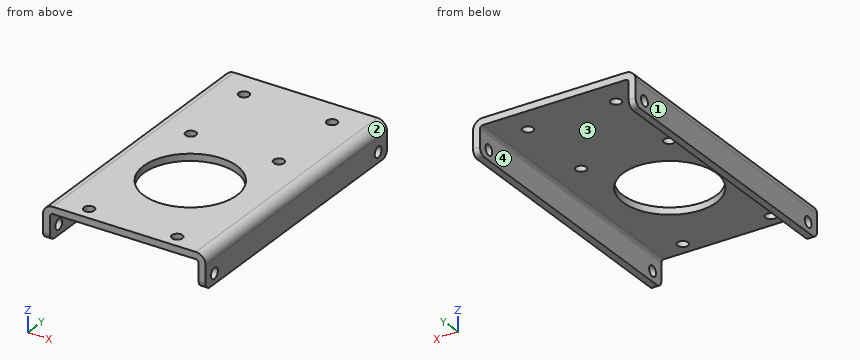
from build123d import *

# Parameters (mm, degrees)
SKETCH1_W                      = 76.2
SKETCH1_H                      = 130.175
BASE_FLANGE1_DEPTH             = 3.2639
EDGE_FLANGE1_STRIP_W           = 15.5956
EDGE_FLANGE1_STRIP_H           = 3.2639
EDGE_FLANGE1_STRIP_CUT_DEPTH   = 130.175
EDGE_FLANGE1_STRIP_2_W         = 15.5956
EDGE_FLANGE1_STRIP_2_H         = 3.2639
EDGE_FLANGE1_STRIP_CUT_2_DEPTH = 130.175
EDGE_FLANGE1_DEPTH             = 130.175
EDGE_FLANGE1_BEND_DEPTH        = 130.175
F_10_0_1935_DIAMETER_HOLE1_D   = 4.9149
SKETCH32_R                     = 21.87575
CUT_EXTRUDE1_DEPTH             = 93.055303045
F_10_0_1935_DIAMETER_HOLE2_D   = 4.9149
FILLET1_R                      = 3.175
F_10_0_1935_DIAMETER_HOLE3_D   = 4.9149


# Sheet-metal steps are written as plain solids
with BuildPart() as part:
    # Sketch1 → Base-Flange1 (new body)
    with BuildSketch(Plane.XY):
        with Locations((0, 17.758918)):
            Rectangle(SKETCH1_W, SKETCH1_H)
    extrude(amount=-BASE_FLANGE1_DEPTH)

    # Edge-Flange1 strip (across the edge) → Edge-Flange1 strip cut (cut)
    with BuildSketch(Plane(origin=(38.1, 82.846418, -3.2639), x_dir=(-1, 0, 0), z_dir=(0, -1, 0))):
        with Locations((-3.2639, -1.63195)):
            Rectangle(EDGE_FLANGE1_STRIP_W, EDGE_FLANGE1_STRIP_H)
    extrude(amount=EDGE_FLANGE1_STRIP_CUT_DEPTH, mode=Mode.SUBTRACT)

    # Edge-Flange1 strip 2 (across the edge) → Edge-Flange1 strip cut 2 (cut)
    with BuildSketch(Plane(origin=(-38.1, -47.328582, -3.2639), x_dir=(1, 0, 0), z_dir=(0, 1, 0))):
        with Locations((-3.2639, -1.63195)):
            Rectangle(EDGE_FLANGE1_STRIP_2_W, EDGE_FLANGE1_STRIP_2_H)
    extrude(amount=EDGE_FLANGE1_STRIP_CUT_2_DEPTH, mode=Mode.SUBTRACT)

    # Edge-Flange1 section (across the edge) → Edge-Flange1 (add)
    with BuildSketch(Plane(origin=(38.1, 82.846418, -3.2639), x_dir=(-1, 0, 0), z_dir=(0, -1, 0))):
        with BuildLine():
            Line((0, 1.27), (0, 12.6111))
            Line((0, 12.6111), (3.2639, 12.6111))
            Line((3.2639, 12.6111), (3.2639, 1.27))
            ThreePointArc((3.2639, 1.27), (3.635874388, 0.371974388), (4.5339, 0))
            Line((4.5339, 0), (4.5339, -3.2639))
            ThreePointArc((4.5339, -3.2639), (1.327948565, -1.935951435), (0, 1.27))
        make_face()
    extrude(amount=EDGE_FLANGE1_DEPTH)

    # Edge-Flange1 section 2 (across the edge) → Edge-Flange1 bend (add)
    with BuildSketch(Plane(origin=(-38.1, -47.328582, -3.2639), x_dir=(1, 0, 0), z_dir=(0, 1, 0))):
        with BuildLine():
            Line((0, 1.27), (0, 12.6111))
            Line((0, 12.6111), (3.2639, 12.6111))
            Line((3.2639, 12.6111), (3.2639, 1.27))
            ThreePointArc((3.2639, 1.27), (3.635874388, 0.371974388), (4.5339, 0))
            Line((4.5339, 0), (4.5339, -3.2639))
            ThreePointArc((4.5339, -3.2639), (1.327948565, -1.935951435), (0, 1.27))
        make_face()
    extrude(amount=EDGE_FLANGE1_BEND_DEPTH)

    # #10 (0.1935) Diameter Hole1 (through all)
    with Locations(Plane(origin=(38.1, 0, 0), x_dir=(0, 0, -1), z_dir=(1, 0, 0))):
        with Locations((11.1125, 76.496418), (11.1125, -40.978582)):
            Hole(F_10_0_1935_DIAMETER_HOLE1_D / 2)

    # Sketch32 → Cut-Extrude1 (cut, through all)
    with BuildSketch(Plane(origin=(0, 0, -3.2639), x_dir=(-1, 0, 0), z_dir=(0, 0, -1))):
        Circle(SKETCH32_R)
    extrude(amount=-CUT_EXTRUDE1_DEPTH, mode=Mode.SUBTRACT)

    # #10 (0.1935) Diameter Hole2 (through all)
    with Locations(Plane.XY):
        with Locations((-20.6375, -40.978582), (20.6375, -40.978582)):
            Hole(F_10_0_1935_DIAMETER_HOLE2_D / 2)

    # Fillet1
    fillet1_edges = [part.edges().sort_by_distance(p)[0] for p in [
        (36.46805, 82.846418, -15.875),
        (36.46805, -47.328582, -15.875),
        (-36.46805, -47.328582, -15.875),
        (-36.46805, 82.846418, -15.875),
    ]]
    fillet(fillet1_edges, radius=FILLET1_R)

    # #10 (0.1935) Diameter Hole3 (through all)
    with Locations(Plane.XY):
        with Locations((-20.6375, 70.146418), (20.6375, 70.146418), (20.6375, 32.046418), (-20.6375, 32.046418)):
            Hole(F_10_0_1935_DIAMETER_HOLE3_D / 2)


solid = part.part
CAD build for the part. Positions are in the model's coordinates, mm. Face numbers are marked on the shaded views. Coordinates: 2 decimals unless noted, no trailing zeros. Order: outer loops, then holes, each group sorted by start corner. A loop starts at its lowest first (then second) coordinate and runs counter-clockwise, first axis right, second up. Notation, with made-up numbers: (-2, -20) -> (6, -20) arc R32 ccw to (6, 7) -> close; hole circle Ø8 at (59.25, 80). An arc over 180 degrees is marked (long way). Answer in a Markdown table with one row per item.
1) Mould opens along X. For the marked faces 1, 2, 3 and 4 say: pulls with the +X half, pulls with the -X half, needs draft (parallel to the pull), parting line crosses it, or undercut.
Check values:
| item | result |
|---|---|
| face 1 | pulls with the -X half |
| face 2 | pulls with the +X half |
| face 3 | undercut |
| face 4 | undercut |
2) Flat gauge pins, fed straight in: P1, Ø4, axis at x = 20.64, y = -40.98, coming from the -Z side; P2, Ø20, axis at x = -16.5, y = 42, coming from the -Z side; P3, Ø8, axis at x = -7.5, y = 65, coming from the +Z side. Where does each tip first touch, or does it go through?
Check values:
| item | result |
|---|---|
| P1 | through |
| P2 | z = -3.26 |
| P3 | z = 0 |
3) Band-saw the part on A-A (x = 0). List the corners of the cut face in (y, z), and give its area (3 significant figures).
Check values:
| item | result |
|---|---|
| outline | (-47.33, -3.26) -> (-21.88, -3.26) -> (-21.88, 0) -> (-47.33, 0) -> close; (21.88, -3.26) -> (82.85, -3.26) -> (82.85, 0) -> (21.88, 0) -> close |
| area | 282 mm2 |
4) Band-saw the part on C-C (z = -10). List the corners of the cut face in (x, y), and give its area (3 significant figures).
Check values:
| item | result |
|---|---|
| outline | (-38.1, -47.33) -> (-34.84, -47.33) -> (-34.84, -43.17) -> (-38.1, -43.17) -> close; (-38.1, -38.79) -> (-34.84, -38.79) -> (-34.84, 74.31) -> (-38.1, 74.31) -> close; (-38.1, 78.69) -> (-34.84, 78.69) -> (-34.84, 82.85) -> (-38.1, 82.85) -> close; (34.84, -47.33) -> (38.1, -47.33) -> (38.1, -43.17) -> (34.84, -43.17) -> close; (34.84, -38.79) -> (38.1, -38.79) -> (38.1, 74.31) -> (34.84, 74.31) -> close; (34.84, 78.69) -> (38.1, 78.69) -> (38.1, 82.85) -> (34.84, 82.85) -> close |
| area | 793 mm2 |
5) Band-saw the part on B-B (y = 0). List the corners of the cut face in (x, z) (3 decimals).
Check values:
| item | result |
|---|---|
| outline | (-38.1, -15.875) -> (-34.836, -15.875) -> (-34.836, -4.534) arc R1.27 cw to (-33.566, -3.264) -> (-21.876, -3.264) -> (-21.876, 0) -> (-33.566, 0) arc R4.534 ccw to (-38.1, -4.534) -> close; (21.876, -3.264) -> (33.566, -3.264) arc R1.27 cw to (34.836, -4.534) -> (34.836, -15.875) -> (38.1, -15.875) -> (38.1, -4.534) arc R4.534 ccw to (33.566, 0) -> (21.876, 0) -> close |
6) Drill centre lines: line 1 (Y direction, x = 35, z = -11.5); line 2 (X direction, y = 7, z = -6.25); line 3 (Z direction, x = 30, y = 25). Where is each one in solid material? Low to high.
Check values:
| item | result |
|---|---|
| line 1 | -47.33 to -43.41, -38.55 to 74.07, 78.92 to 82.85 |
| line 2 | -38.1 to -34.84, 34.84 to 38.1 |
| line 3 | -3.26 to 0 |
7) Band-saw the part on D-D (y = 59). List the corners of the cut face in (x, z) (3 decimals), and give its area (3 significant figures).
Check values:
| item | result |
|---|---|
| outline | (-38.1, -15.875) -> (-34.836, -15.875) -> (-34.836, -4.534) arc R1.27 cw to (-33.566, -3.264) -> (33.566, -3.264) arc R1.27 cw to (34.836, -4.534) -> (34.836, -15.875) -> (38.1, -15.875) -> (38.1, -4.534) arc R4.534 ccw to (33.566, 0) -> (-33.566, 0) arc R4.534 ccw to (-38.1, -4.534) -> close |
| area | 323 mm2 |
